from build123d import *

# Parameters (mm, degrees)
PAD_DEPTH    = 2
FILLET_R     = 1
SKETCH001_W  = 3.5
SKETCH001_H  = 1
POCKET_DEPTH = 1.5
PAD001_DEPTH = 2
FILLET001_R  = 0.5


with BuildPart() as part:
    # Sketch → Pad (new body)
    with BuildSketch(Plane.XY):
        Polygon((-18.5, 2.5), (-8.5, 2.5), (-8.5, 0.5), (-5, 0.5), (-5, 2.5), (5, 2.5), (5, 0.5), (8.5, 0.5), (8.5, 2.5), (18.5, 2.5), (18.5, -2.5), (8.5, -2.5), (8.5, -0.5), (5, -0.5), (5, -2.5), (-5, -2.5), (-5, -0.5), (-8.5, -0.5), (-8.5, -2.5), (-18.5, -2.5), align=None)
    extrude(amount=PAD_DEPTH)

    # Fillet
    fillet_edges = [part.edges().sort_by_distance(p)[0] for p in [
        (-18.5, 2.5, 1),
        (-5, 2.5, 1),
        (8.5, 2.5, 1),
        (-18.5, -2.5, 1),
        (-5, -2.5, 1),
        (8.5, -2.5, 1),
        (-8.5, 2.5, 1),
        (-8.5, -2.5, 1),
        (5, 2.5, 1),
        (5, -2.5, 1),
        (18.5, 2.5, 1),
        (18.5, -2.5, 1),
    ]]
    fillet(fillet_edges, radius=FILLET_R)

    # Sketch001 → Pocket (cut)
    with BuildSketch(Plane.XY.offset(2)):
        with Locations((-6.75, 0)):
            Rectangle(SKETCH001_W, SKETCH001_H)
        with Locations((6.75, 0)):
            Rectangle(SKETCH001_W, SKETCH001_H)
    extrude(amount=-POCKET_DEPTH, mode=Mode.SUBTRACT)

    # Sketch002 → Pad001 (new body)
    with BuildSketch(Plane.XY.offset(2)):
        with BuildLine():
            ThreePointArc((-15.5, 1.8), (-17.3, 0), (-15.5, -1.8))
            Line((-15.5, -1.8), (-11.5, -1.8))
            ThreePointArc((-11.5, -1.8), (-9.7, 0), (-11.5, 1.8))
            Line((-15.5, 1.8), (-11.5, 1.8))
        make_face()
        with BuildLine():
            ThreePointArc((-2, 1.8), (-3.8, 0), (-2, -1.8))
            Line((-2, -1.8), (2, -1.8))
            ThreePointArc((2, -1.8), (3.8, 0), (2, 1.8))
            Line((-2, 1.8), (2, 1.8))
        make_face()
        with BuildLine():
            ThreePointArc((11.5, 1.8), (9.7, 0), (11.5, -1.8))
            Line((15.5, -1.8), (11.5, -1.8))
            ThreePointArc((15.5, -1.8), (17.3, 0), (15.5, 1.8))
            Line((11.5, 1.8), (15.5, 1.8))
        make_face()
    extrude(amount=PAD001_DEPTH)

    # Fillet001
    fillet001_edges = [part.edges().sort_by_distance(p)[0] for p in [
        (-17.3, 0, 4),
        (-13.5, -1.8, 4),
        (-9.7, 0, 4),
        (-13.5, 1.8, 4),
        (-3.8, 0, 4),
        (0, -1.8, 4),
        (3.8, 0, 4),
        (0, 1.8, 4),
        (17.3, 0, 4),
        (13.5, 1.8, 4),
        (9.7, 0, 4),
        (13.5, -1.8, 4),
    ]]
    fillet(fillet001_edges, radius=FILLET001_R)


solid = part.part
Work out the finished part from the listing and answer in its coordinate system (mm). A direction names the side the tool comes from. Give positions to 0.01 mm unless a question says otherwise; leave off trailing zeros. Loops run counter-clockwise (first coordinate to the right, second up) from the corner with the lowest first, then second, coordinate; pieces in that order, holes last. Notation, with made-up numbers: (36, 52.5) -> (52, 52.5) arc R35 cw to (52, 86.5) -> close; hole circle Ø10 at (80.25, 59.25). An arc over 180 degrees is marked (long way). Use a Markdown table: item, result. Add a question column.
1. For faces 1 (the flat face through (-14, 1.8, 3)), 2 (the cylindrical face through (-17.3, 0, 2.7)), 3 (the cylindrical face through (-9.7, 0, 2.7)), determine the directions among +Z, -Z, +X, -X, +Y, -Y from which every point of the face is accessible in a straight line to the end or side of a thin tool.
2. Section B-B on x = -0.5 is taken. Determine the outline of the cut face in (y, z), and give its area (3 significant figures).
3. Flat-ended cylindrical pins translate along their axes: pin 1 Ø0.6 at (x, z) = (-7, 0) entering from -Y; pin 2 Ø0.8 at (x, y) = (7, 0) entering from +Z; pin 3 Ø1.6 at (x, z) = (14.5, 3) entering from -Y. Find the tip coordinate at first contact, or state that the pin passes through.
4. Find the intervals of material crossed by probe 1 along X at (y, z) = (-0.1, 0.6); probe 2 along X at (y, z) = (-0.9, 2.6); probe 3 along Z at (x, y) = (15, -2.3), in increasing order.
5. Section A-A on z = 1.55 is taken. Determine the outline of the cut face in (x, y), and give its area (3 significant figures).
6. Section D-D on x = -8 is taken. Determine the outline of the cut face in (y, z), and give its area (3 significant figures).
7. Determine the mould class of faces 4 (the flat face through (8.5, 0, 1)), 5 (the flat face through (14, -2.5, 1)), 6 (the cylindrical face through (17.3, 0, 2.7)) for opening direction X: released by +X, released by -X, zero draft, split by the parting line, or undercut.
Results below:
| question | item | result |
|---|---|---|
| 1 | face 1 | +Z, +X, -X, +Y |
| 1 | face 2 | +Z, -X |
| 1 | face 3 | +Z |
| 2 | outline | (-2.5, 0) -> (2.5, 0) -> (2.5, 2) -> (1.8, 2) -> (1.8, 3.5) arc R0.5 ccw to (1.3, 4) -> (-1.3, 4) arc R0.5 ccw to (-1.8, 3.5) -> (-1.8, 2) -> (-2.5, 2) -> close |
| 2 | area | 17.1 mm^2 |
| 3 | pin 1 | stops at y = -0.5 |
| 3 | pin 2 | stops at z = 0.5 |
| 3 | pin 3 | stops at y = -1.8 |
| 4 | probe 1 | x = -18.5 to -8.5, -5 to 5, 8.5 to 18.5 |
| 4 | probe 2 | x = -17.06 to -9.94, -3.56 to 3.56, 9.94 to 17.06 |
| 4 | probe 3 | z = 0 to 2 |
| 5 | outline | (-18.5, -1.5) arc R1 ccw to (-17.5, -2.5) -> (-9.5, -2.5) arc R1 ccw to (-8.5, -1.5) -> (-8.5, 1.5) arc R1 ccw to (-9.5, 2.5) -> (-17.5, 2.5) arc R1 ccw to (-18.5, 1.5) -> close; (-5, -1.5) arc R1 ccw to (-4, -2.5) -> (4, -2.5) arc R1 ccw to (5, -1.5) -> (5, 1.5) arc R1 ccw to (4, 2.5) -> (-4, 2.5) arc R1 ccw to (-5, 1.5) -> close; (8.5, -1.5) arc R1 ccw to (9.5, -2.5) -> (17.5, -2.5) arc R1 ccw to (18.5, -1.5) -> (18.5, 1.5) arc R1 ccw to (17.5, 2.5) -> (9.5, 2.5) arc R1 ccw to (8.5, 1.5) -> close |
| 5 | area | 147 mm^2 |
| 6 | outline | (-0.5, 0) -> (0.5, 0) -> (0.5, 0.5) -> (-0.5, 0.5) -> close |
| 6 | area | 0.500 mm^2 |
| 7 | face 4 | undercut |
| 7 | face 5 | zero draft |
| 7 | face 6 | released by +X |
